from build123d import *

# Parameters (mm, degrees)
SKETCH1_R           = 4.445
SKETCH1_R_2         = 17.4625
BOSS_EXTRUDE1_DEPTH = 6.35


with BuildPart() as part:
    # Sketch1 → Boss-Extrude1 (new body)
    with BuildSketch(Plane(origin=(0, 0, 0), x_dir=(1, 0, 0), z_dir=(0, 1, 0))):
        with BuildLine():
            ThreePointArc((-19.05, -50.8), (0, -69.85), (19.05, -50.8))
            Line((19.05, -50.8), (25.4, 0))
            Line((25.4, 0), (19.05, 50.8))
            ThreePointArc((19.05, 50.8), (0, 69.85), (-19.05, 50.8))
            Line((-19.05, 50.8), (-25.4, 0))
            Line((-25.4, 0), (-19.05, -50.8))
        make_face()
        with Locations((0, -50.8)):
            Circle(SKETCH1_R, mode=Mode.SUBTRACT)
        Circle(SKETCH1_R_2, mode=Mode.SUBTRACT)
        with Locations((0, 50.8)):
            Circle(SKETCH1_R, mode=Mode.SUBTRACT)
    extrude(amount=BOSS_EXTRUDE1_DEPTH)


solid = part.part
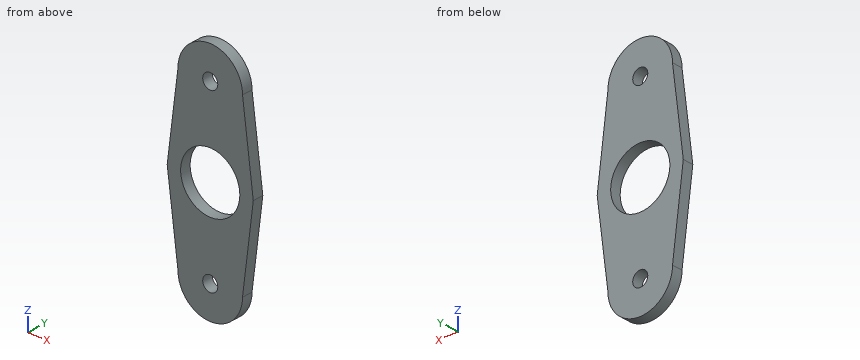
Source: CAD feature listing. Evaluate the final solid. Frame: model axes, mm. Round coordinates to 2 decimals unless told otherwise and drop trailing zeros. Loops run counter-clockwise (first coordinate to the right, second up) from the corner with the lowest first, then second, coordinate; pieces in that order, holes last. Notation, with made-up numbers: (79, -3.75) - (98, -3.75) arc R7 cw to (98, 8.25) - close; hole circle Ø10 at (56, 21.5). An arc over 180 degrees is marked (long way). Write item = value, one per line. Start each with the question number.
Item 1: Material intervals for line 1 (X direction, y = 2.5, z = -50.8) (3 decimals); line 2 (Z direction, x = -1.5, y = 1.5); line 3 (Z direction, x = -8, y = 0.5), sorted ascending.
Item 2: Section query D-D on z = -33. Output: boundary loops of the cut face in (x, y) (3 decimals), plus the area to 3 significant figures.
Item 3: First-contact query: pin 1 Ø10 at (x, z) = (0, -50.8) entering from -Y; pin 2 Ø12 at (x, z) = (-7, 7.5) entering from +Y; pin 3 Ø2 at (y, z) = (4, -31) entering from +X; pin 4 Ø1.5 at (x, y) = (-1.5, 3) entering from -Z. Flat tips, straight axial feed; report the tip coordinate or a pass-through.
Item 4: Section query A-A on x = 0. Count the separate pieces of the cut face and the enclosed holes in it, plus the area to 3 significant figures.
Item 5: Section query C-C on z = 20. Output: boundary loops of the cut face in (x, y), plus the area to 3 significant figures.
Item 6: Section query B-B on z = 5.5. Output: boundary loops of the cut face in (x, y).
Results list:
q1.line_1 = -19.05 to -4.445, 4.445 to 19.05
q1.line_2 = -69.79 to -54.98, -46.62 to -17.4, 17.4 to 46.62, 54.98 to 69.79
q1.line_3 = -68.09 to -15.52, 15.52 to 68.09
q2.outline = (-21.275, 0) - (21.275, 0) - (21.275, 6.35) - (-21.275, 6.35) - close
q2.area = 270 mm²
q3.pin_1 = 0
q3.pin_2 = through
q3.pin_3 = 21.65
q3.pin_4 = -69.84
q4.separate_pieces = 4
q4.enclosed_holes = 0
q4.area = 552 mm²
q5.outline = (-22.9, 0) - (22.9, 0) - (22.9, 6.35) - (-22.9, 6.35) - close
q5.area = 291 mm²
q6.outline = (-24.71, 0) - (-16.57, 0) - (-16.57, 6.35) - (-24.71, 6.35) - close; (16.57, 0) - (24.71, 0) - (24.71, 6.35) - (16.57, 6.35) - close
